Geometry check sheet. Reference: the model listing, model coordinates, mm. A direction names the side the tool comes from. Round coordinates to 2 decimals unless told otherwise and drop trailing zeros. Write each loop counter-clockwise with the first axis right and the second up, starting at its lowest first coordinate (ties: lowest second). Pieces come first, ordered by that corner, then holes.
from build123d import *

# Parameters (mm, degrees)
SKETCH1_R           = 57.5
BOSS_EXTRUDE1_DEPTH = 15
SKETCH2_R           = 50
CUT_EXTRUDE1_DEPTH  = 11
SKETCH3_R           = 1.75
SKETCH3_R_2         = 15
CUT_EXTRUDE2_DEPTH  = 15
CUT_EXTRUDE3_START  = -15
CUT_EXTRUDE3_DEPTH  = 15
CHAMFER1_SIZE       = 7
SKETCH5_R           = 3.25
CUT_EXTRUDE4_DEPTH  = 7


with BuildPart() as part:
    # Sketch1 → Boss-Extrude1 (new body)
    with BuildSketch(Plane(origin=(0, 0, 0), x_dir=(1, 0, 0), z_dir=(0, 1, 0))):
        with Locations(Location((0, 0, 0), (0, 0, 270))):
            Circle(SKETCH1_R)
    extrude(amount=BOSS_EXTRUDE1_DEPTH)

    # Sketch2 → Cut-Extrude1 (cut)
    with BuildSketch(Plane.XZ):
        with Locations(Location((0, 0, 0), (0, 0, 270))):
            Circle(SKETCH2_R)
    extrude(amount=-CUT_EXTRUDE1_DEPTH, mode=Mode.SUBTRACT)

    # Sketch3 → Cut-Extrude2 (cut)
    with BuildSketch(Plane(origin=(0, 15, 0), x_dir=(1, 0, 0), z_dir=(0, 1, 0))):
        with Locations(Location((0, 54, 0), (0, 0, 270))):
            Circle(SKETCH3_R)
        with Locations(Location((27, 46.765371804, 0), (0, 0, 270))):
            Circle(SKETCH3_R)
        with Locations(Location((46.765371804, 27, 0), (0, 0, 270))):
            Circle(SKETCH3_R)
        with Locations(Location((54, 0, 0), (0, 0, 270))):
            Circle(SKETCH3_R)
        with Locations(Location((46.765371804, -27, 0), (0, 0, 270))):
            Circle(SKETCH3_R)
        with Locations(Location((27, -46.765371804, 0), (0, 0, 270))):
            Circle(SKETCH3_R)
        with Locations(Location((0, -54, 0), (0, 0, 270))):
            Circle(SKETCH3_R)
        with Locations(Location((-27, -46.765371804, 0), (0, 0, 270))):
            Circle(SKETCH3_R)
        with Locations(Location((-46.765371804, -27, 0), (0, 0, 270))):
            Circle(SKETCH3_R)
        with Locations(Location((-54, 0, 0), (0, 0, 270))):
            Circle(SKETCH3_R)
        with Locations(Location((-46.765371804, 27, 0), (0, 0, 270))):
            Circle(SKETCH3_R)
        with Locations(Location((-27, 46.765371804, 0), (0, 0, 270))):
            Circle(SKETCH3_R)
        with Locations(Location((0, 0, 0), (0, 0, 270))):
            Circle(SKETCH3_R_2)
    extrude(amount=-CUT_EXTRUDE2_DEPTH, mode=Mode.SUBTRACT)

    # Sketch4 → Cut-Extrude3 (cut)
    with BuildSketch(Plane(origin=(0, 15, 0), x_dir=(1, 0, 0), z_dir=(0, 1, 0)).offset(CUT_EXTRUDE3_START)):
        with BuildLine():
            Line((25, 25), (40.658639918, 40.658639918))
            ThreePointArc((40.658639918, 40.658639918), (57.5, 0), (40.658639918, -40.658639918))
            Line((40.658639918, -40.658639918), (25, -25))
            Line((25, -25), (25, 25))
        make_face()
    cut_extrude3 = extrude(amount=CUT_EXTRUDE3_DEPTH, mode=Mode.SUBTRACT)

    # Mirror1: Cut-Extrude3 across plane
    add(cut_extrude3.mirror(Plane(origin=(0, 0, 0), x_dir=(0, 0, 1), z_dir=(1, 0, 0))), mode=Mode.SUBTRACT)

    # Chamfer1
    # the kernel refuses this chamfer: 7 mm, written as the material it adds along each edge
    with BuildSketch(Plane(origin=(0, 11, 0), x_dir=(-0.7071067811865476, 0, 0.7071067811865476), z_dir=(-0.7071067811865476, 0, -0.7071067811865476))) as chamfer1_piece_1:
        Polygon((50 - CHAMFER1_SIZE, 0), (50, -CHAMFER1_SIZE), (50, 0), align=None)
    revolve(axis=Axis((0, 11, 0), (0, 1, 0)), revolution_arc=90)
    with BuildSketch(Plane(origin=(0, 11, 0), x_dir=(0.7071067811865475, 0, -0.7071067811865477), z_dir=(0.7071067811865477, 0, 0.7071067811865475))) as chamfer1_piece_2:
        Polygon((50, -CHAMFER1_SIZE), (50 - CHAMFER1_SIZE, 0), (50, 0), align=None)
    revolve(axis=Axis((0, 11, 0), (0, 1, 0)), revolution_arc=90)
    # the kernel refuses this chamfer: 7 mm, written as the material it takes off along each edge
    with BuildSketch(Plane(origin=(0, 15, 0), x_dir=(-0.890570714861766, 0, -0.4548448107108656), z_dir=(-0.4548448107108656, 0, 0.890570714861766))) as chamfer1_2_piece_1:
        Polygon((57.5, CHAMFER1_SIZE), (57.5 - CHAMFER1_SIZE, 0), (57.5, 0), align=None)
    revolve(axis=Axis((0, 15, 0), (0, -1, 0)), revolution_arc=125.890100955, mode=Mode.SUBTRACT)
    with BuildSketch(Plane(origin=(0, 15, 0), x_dir=(0.890570714861766, 0, 0.4548448107108656), z_dir=(0.4548448107108656, 0, -0.890570714861766))) as chamfer1_2_piece_2:
        Polygon((57.5 - CHAMFER1_SIZE, 0), (57.5, CHAMFER1_SIZE), (57.5, 0), align=None)
    revolve(axis=Axis((0, 15, 0), (0, -1, 0)), revolution_arc=125.890100955, mode=Mode.SUBTRACT)

    # Sketch5 → Cut-Extrude4 (cut)
    with BuildSketch(Plane(origin=(0, 15, 0), x_dir=(1, 0, 0), z_dir=(0, 1, 0))):
        with Locations(Location((0, 54, 0), (0, 0, 270))):
            Circle(SKETCH5_R)
        with Locations(Location((27, 46.765371804, 0), (0, 0, 270))):
            Circle(SKETCH5_R)
        with Locations((46.765371804, 27)):
            Circle(SKETCH5_R)
        with Locations((54, 0)):
            Circle(SKETCH5_R)
        with Locations((46.765371804, -27)):
            Circle(SKETCH5_R)
        with Locations(Location((27, -46.765371804, 0), (0, 0, 270))):
            Circle(SKETCH5_R)
        with Locations(Location((0, -54, 0), (0, 0, 270))):
            Circle(SKETCH5_R)
        with Locations(Location((-27, -46.765371804, 0), (0, 0, 270))):
            Circle(SKETCH5_R)
        with Locations((-46.765371804, -27)):
            Circle(SKETCH5_R)
        with Locations((-54, 0)):
            Circle(SKETCH5_R)
        with Locations((-46.765371804, 27)):
            Circle(SKETCH5_R)
        with Locations(Location((-27, 46.765371804, 0), (0, 0, 270))):
            Circle(SKETCH5_R)
    extrude(amount=-CUT_EXTRUDE4_DEPTH, mode=Mode.SUBTRACT)


solid = part.part
1. Section check B-B (x = 0). State how many separate pieces and enclosed holes the cut face has, plus the area to 4 significant figures.
2. Section check A-A (y = 2.25). Record the cut outline in (x, z), plus the area to 3 significant figures.
3. Section check D-D (y = 12.25). Record the cut outline in (x, z), plus the area to 3 significant figures.
4. Scan lines: line 1 along Y through (x, z) = (-24, -6); line 2 along X through (y, z) = (1.75, 46); line 3 along X through (y, z) = (14.75, -20). Record each from-to range of solid material in increasing order.
5. Access from +Z, -Z, +X, -X, +Y, -Y to the whole of each face (thin tool, end or side, straight path). Record for faces 1 (the face through (0, 10, -44)), 2 (the face through (-28, 8, -45)), 3 (the face through (0.632, 3.944, -57.497)).
6. Depth check by flat-ended pin: pin 1 Ø3 at (x, z) = (-27.5, 47) entering from +Y; pin 2 Ø1.2 at (y, z) = (13.5, 3.5) entering from -X; pin 3 Ø8 at (x, y) = (15, 5) entering from +Z. Enter the tip coordinate at first touch or a pass-through.
7. Release check for a two-part mould opening along Z. For faces 4 (the face through (-3, 0, -51)), 5 (the face through (0.98, 10.67, -50.9)), 6 (the face through (8.28, 14.66, -50.16)) record: +Z half, -Z half, draft (parallel to the pull), parting line (faces both ways), or undercut.
8. Section check C-C (z = 27). Record the cut outline in (x, y).
Results below:
1. separate pieces: 4
1. enclosed holes: 0
1. area: 403.5 mm2
2. outline: (-40.66, -40.66) arc R57.5 ccw to (40.66, -40.66) - (35.36, -35.36) arc R50 cw to (-35.36, -35.36) - close; (-40.66, 40.66) - (-35.36, 35.36) arc R50 cw to (35.36, 35.36) - (40.66, 40.66) arc R57.5 ccw to start; hole circle Ø3.5 at (-27, -46.77); hole circle Ø3.5 at (-27, 46.77); hole circle Ø3.5 at (0, -54); hole circle Ø3.5 at (0, 54); hole circle Ø3.5 at (27, -46.77); hole circle Ø3.5 at (27, 46.77)
2. area: 1,210 mm2
3. outline: (-37.65, -37.65) arc R53.25 ccw to (-29.3, -44.47) arc R3.25 cw to (-23.86, -47.61) arc R53.25 ccw to (-3.14, -53.16) arc R3.25 cw to (3.14, -53.16) arc R53.25 ccw to (23.86, -47.61) arc R3.25 cw to (29.3, -44.47) arc R53.25 ccw to (37.65, -37.65) - (25, -25) - (25, 25) - (37.65, 37.65) arc R53.25 ccw to (29.3, 44.47) arc R3.25 cw to (23.86, 47.61) arc R53.25 ccw to (3.14, 53.16) arc R3.25 cw to (-3.14, 53.16) arc R53.25 ccw to (-23.86, 47.61) arc R3.25 cw to (-29.3, 44.47) arc R53.25 ccw to (-37.65, 37.65) - (-25, 25) - (-25, -25) - close; hole circle Ø30 at (0, 0)
3. area: 4,930 mm2
4. line 1: y = 11 to 15
4. line 2: x = -34.5 to -28.57, -25.43 to -19.6, 19.6 to 25.43, 28.57 to 34.5
4. line 3: x = -25 to 25
5. face 1: -Y
5. face 2: +Y
5. face 3: -Z, +Y, -Y
6. pin 1: stops at y = 8
6. pin 2: stops at x = -25
6. pin 3: stops at z = 56.44
7. face 4: draft
7. face 5: undercut
7. face 6: -Z half
8. outline: (-27, 11) - (27, 11) - (27, 15) - (-27, 15) - close
